Autodesk Inventor part; units mm, degrees
ref_plane "YZ Plane" through (0, 0, 0) normal (1, 0, 0) x (0, 1, 0)
ref_plane "XZ Plane" through (0, 0, 0) normal (0, 1, 0) x (-1, 0, 0)
ref_plane "XY Plane" through (0, 0, 0) normal (0, 0, 1) x (1, 0, 0)
sketch "Sketch1" plane through (0, 0, 0) normal (1, 0, 0) x (0, 1, 0)
  line L0 (0, 0) -> (3.175, 0)
  line L1 (3.175, 0) -> (3.175, -25.4)
  line L2 (3.175, -25.4) -> (-22.225, -25.4)
  line L3 (-22.225, -25.4) -> (-22.225, -22.225)
  line L4 (-22.225, -22.225) -> (0, -22.225)
  line L5 (0, -22.225) -> (0, 0)
  dimension "d0" = 3.175
  dimension "d1" = 3.175
  dimension "d2" = 25.4
  dimension "d3" = 25.4
extrude "Extrusion1" add sketch "Sketch1" along normal blind 25.4
sketch "Sketch2" plane through (0, 0, 0) normal (-1, 0, 0) x (0, 0, 1)
  line L0 (-25.4, -22.225) -> (-25.4, 3.175)
  line L1 (-25.4, 3.175) -> (0, 3.175)
  line L2 (0, 3.175) -> (0, -22.225)
  line L3 (0, -22.225) -> (-25.4, -22.225)
  line L4 (-25.4, -22.225) -> (-25.4, 3.175)
  line L5 (-25.4, -22.225) -> (-22.225, -22.225)
  point P0 (0, 0)
extrude "Extrusion2" add sketch "Sketch2" against normal blind 3.175
properties part number "gusset_plate_corner"
Verification items for the finished model (mm, model axes). A direction names the side the tool comes from. Round coordinates to 2 decimals unless told otherwise and drop trailing zeros. Order: outer loops, then holes, each group sorted by start corner. A loop starts at its lowest first (then second) coordinate and runs counter-clockwise, first axis right, second up.
1) Cross-section at A-A, the plane z = -6.25. Record the cut outline in (x, y) (3 decimals), plus the area to 3 significant figures.
Geometry says:
outline: (0, -22.225) - (3.175, -22.225) - (3.175, 0) - (25.4, 0) - (25.4, 3.175) - (0, 3.175) - close
area: 151 mm2
2) Cross-section at B-B, the plane x = 21. Record the cut outline in (y, z) (3 decimals), plus the area to 3 significant figures.
Geometry says:
outline: (-22.225, -25.4) - (3.175, -25.4) - (3.175, 0) - (0, 0) - (0, -22.225) - (-22.225, -22.225) - close
area: 151 mm2
3) Material ranges on line 1 (Z direction, x = 6.75, y = -11.5) (3 decimals); line 2 (Y direction, x = 17, z = -19.75) (3 decimals), recorded low to high.
Geometry says:
line 1: z = -25.4 to -22.225
line 2: y = 0 to 3.175
4) Depth check by flat-ended pin: pin 1 (6 mm diameter, centred on y = -4, z = -7, fed in from +X) (3 decimals); pin 2 (6.5 mm diameter, centred on x = 13, z = -9.5, fed in from -Y). Enter the tip coordinate at first touch or a pass-through.
Geometry says:
pin 1: stops at x = 3.175
pin 2: stops at y = 0
5) Tool access check on faces 1 (the flat face through (14, -11, -22.225)), 2 (the flat face through (2, -5, 0)). Record the directions out of +Z, -Z, +X, -X, +Y, -Y that give a thin tool (end or side, any length) a straight path to the whole face; none if there is none.
Geometry says:
face 1: +Z, +X, -Y
face 2: +Z, +X, -X, +Y, -Y
